Here's how the part is built. I have some questions about the finished solid (model axes, mm). A direction names the side the tool comes from. Coordinates: 2 decimals unless noted, no trailing zeros. Loops run counter-clockwise (first coordinate to the right, second up) from the corner with the lowest first, then second, coordinate; pieces in that order, holes last. Notation, with made-up numbers: (78, 20) - (117, 20) arc R18 ccw to (117, 51) - close; hole circle Ø7 at (-21, 80.25). An arc over 180 degrees is marked (long way). Use a Markdown table: item, result.
```python
from build123d import *

# Parameters (mm, degrees)
SKETCH1_W           = 335.5
SKETCH1_H           = 193
BOSS_EXTRUDE1_DEPTH = 1.5
BOSS_EXTRUDE2_DEPTH = 2
BOSS_EXTRUDE3_DEPTH = 4
SKETCH5_R           = 4
CUT_EXTRUDE1_DEPTH  = 4
SKETCH6_R           = 1.9
CUT_EXTRUDE2_DEPTH  = 14


with BuildPart() as part:
    # Sketch1 → Boss-Extrude1 (new body)
    with BuildSketch(Plane.XY):
        Rectangle(SKETCH1_W, SKETCH1_H)
    extrude(amount=BOSS_EXTRUDE1_DEPTH)

    # Sketch2 → Boss-Extrude2 (add)
    with BuildSketch(Plane.XY.offset(1.5)):
        with BuildLine():
            Line((-153.75, -90.5), (-153.75, -94.5))
            Line((-153.75, -94.5), (-6, -94.5))
            Line((-6, -94.5), (-6, -88.4))
            ThreePointArc((-6, -88.4), (-4.271930009, -84.228069991), (-0.1, -82.5))
            Line((-0.1, -82.5), (0.1, -82.5))
            ThreePointArc((0.1, -82.5), (4.271930009, -84.228069991), (6, -88.4))
            Line((6, -88.4), (6, -94.5))
            Line((6, -94.5), (153.75, -94.5))
            Line((153.75, -94.5), (153.75, -90.5))
            ThreePointArc((153.75, -90.5), (156.093145751, -84.843145751), (161.75, -82.5))
            Line((161.75, -82.5), (165.75, -82.5))
            Line((165.75, -82.5), (165.75, 82.5))
            Line((165.75, 82.5), (161.75, 82.5))
            ThreePointArc((161.75, 82.5), (156.093145751, 84.843145751), (153.75, 90.5))
            Line((153.75, 90.5), (153.75, 94.5))
            Line((153.75, 94.5), (6, 94.5))
            Line((6, 94.5), (-6, 94.5))
            Line((-6, 94.5), (-153.75, 94.5))
            Line((-153.75, 94.5), (-165.75, 94.5))
            Line((-165.75, 94.5), (-165.75, 82.5))
            Line((-165.75, 82.5), (-165.75, -82.5))
            Line((-165.75, -82.5), (-161.75, -82.5))
            ThreePointArc((-161.75, -82.5), (-156.093145751, -84.843145751), (-153.75, -90.5))
        make_face()
    extrude(amount=BOSS_EXTRUDE2_DEPTH)

    # Sketch4 → Boss-Extrude3 (add)
    with BuildSketch(Plane.XY.offset(1.5)):
        with BuildLine():
            Line((-165.75, -82.5), (-165.75, -94.5))
            Line((-165.75, -94.5), (-153.75, -94.5))
            Line((-153.75, -94.5), (-153.75, -90.5))
            ThreePointArc((-153.75, -90.5), (-156.093145751, -84.843145751), (-161.75, -82.5))
            Line((-161.75, -82.5), (-165.75, -82.5))
        make_face()
        with BuildLine():
            Line((-6, -94.5), (6, -94.5))
            Line((6, -94.5), (6, -88.4))
            ThreePointArc((6, -88.4), (4.271930009, -84.228069991), (0.1, -82.5))
            Line((0.1, -82.5), (-0.1, -82.5))
            ThreePointArc((-0.1, -82.5), (-4.271930009, -84.228069991), (-6, -88.4))
            Line((-6, -88.4), (-6, -94.5))
        make_face()
        with BuildLine():
            Line((153.75, -94.5), (165.75, -94.5))
            Line((165.75, -94.5), (165.75, -82.5))
            Line((165.75, -82.5), (161.75, -82.5))
            ThreePointArc((161.75, -82.5), (156.093145751, -84.843145751), (153.75, -90.5))
            Line((153.75, -90.5), (153.75, -94.5))
        make_face()
        with BuildLine():
            Line((165.75, 94.5), (165.75, 82.5))
            Line((165.75, 82.5), (161.75, 82.5))
            ThreePointArc((161.75, 82.5), (156.093145751, 84.843145751), (153.75, 90.5))
            Line((153.75, 90.5), (153.75, 94.5))
            Line((153.75, 94.5), (165.75, 94.5))
        make_face()
        with BuildLine():
            Line((-165.75, 24.6), (-165.75, 12.6))
            Line((-165.75, 12.6), (-159.65, 12.6))
            ThreePointArc((-159.65, 12.6), (-153.65, 18.6), (-159.65, 24.6))
            Line((-159.65, 24.6), (-165.75, 24.6))
        make_face()
        with BuildLine():
            Line((-83.85, 94.5), (-95.85, 94.5))
            Line((-95.85, 94.5), (-95.85, 88.4))
            ThreePointArc((-95.85, 88.4), (-94.121930009, 84.228069991), (-89.95, 82.5))
            Line((-89.95, 82.5), (-89.75, 82.5))
            ThreePointArc((-89.75, 82.5), (-85.578069991, 84.228069991), (-83.85, 88.4))
            Line((-83.85, 88.4), (-83.85, 94.5))
        make_face()
        with BuildLine():
            Line((46.25, 94.5), (34.25, 94.5))
            Line((34.25, 94.5), (34.25, 88.4))
            ThreePointArc((34.25, 88.4), (40.25, 82.4), (46.25, 88.4))
            Line((46.25, 88.4), (46.25, 94.5))
        make_face()
    extrude(amount=BOSS_EXTRUDE3_DEPTH)

    # Sketch5 → Cut-Extrude1 (cut)
    with BuildSketch(Plane(origin=(0, 0, 0), x_dir=(-1, 0, 0), z_dir=(0, 0, -1))):
        with Locations((-159.75, 88.5)):
            Circle(SKETCH5_R)
        with Locations((0, -88.5)):
            Circle(SKETCH5_R)
        with Locations((159.75, -88.5)):
            Circle(SKETCH5_R)
        with Locations((-159.75, -88.5)):
            Circle(SKETCH5_R)
        with Locations((89.75, 88.5)):
            Circle(SKETCH5_R)
        with Locations((-40.25, 88.4)):
            Circle(SKETCH5_R)
        with Locations((159.75, 18.6)):
            Circle(SKETCH5_R)
    extrude(amount=-CUT_EXTRUDE1_DEPTH, mode=Mode.SUBTRACT)

    # Sketch6 → Cut-Extrude2 (cut)
    with BuildSketch(Plane(origin=(0, 0, 0), x_dir=(-1, 0, 0), z_dir=(0, 0, -1))):
        with Locations((-159.75, -88.5)):
            Circle(SKETCH6_R)
        with Locations((0, -88.5)):
            Circle(SKETCH6_R)
        with Locations((159.75, -88.5)):
            Circle(SKETCH6_R)
        with Locations((-159.75, 88.5)):
            Circle(SKETCH6_R)
        with Locations((89.75, 88.5)):
            Circle(SKETCH6_R)
        with Locations((159.75, 18.6)):
            Circle(SKETCH6_R)
        with Locations((-40.25, 88.4)):
            Circle(SKETCH6_R)
    extrude(amount=-CUT_EXTRUDE2_DEPTH, mode=Mode.SUBTRACT)


solid = part.part
```
Q1. Please list where these lines run through material, in increasing order: L1, parallel to Y at x = -159.75, z = 2.7; L2, parallel to Y at x = 40.25, z = 2.9; L3, parallel to Y at x = 159.75, z = 5.25. Write a range as from..to.
Check values:
| item | result |
|---|---|
| L1 | -94.5..-92.5, -84.5..14.6, 22.6..94.5 |
| L2 | -94.5..84.4, 92.4..94.5 |
| L3 | -94.5..-90.4, -86.6..-82.75, 82.75..86.6, 90.4..94.5 |
Q2. I want a section at C-C, the plane x = -128.5. Write out the boundary of the cut face in (y, z).
Check values:
| item | result |
|---|---|
| outline | (-96.5, 0) - (96.5, 0) - (96.5, 1.5) - (94.5, 1.5) - (94.5, 3.5) - (-94.5, 3.5) - (-94.5, 1.5) - (-96.5, 1.5) - close |
Q3. Which directions (+Z, -Z, +X, -X, +Y, -Y) give clear straight access to the entire face, cutting with the end or side of a thin tool? Please do faces 5 (the face through (-85.624, 84.182, 4.486)), 6 (the face through (-161.596, -92.049, 1.972)), 7 (the face through (156.156, 84.781, 4.486)).
Check values:
| item | result |
|---|---|
| face 5 | +Z, -Y |
| face 6 | -Z |
| face 7 | +Z |
Q4. If we mould it in two halves opening along Y, with no side actions, what happens to faces 1 (the face through (-163, -88, 5.5)), 2 (the face through (4.318, -84.274, 4.486)), 3 (the face through (-2, -89, 4)), 4 (the face through (-94.168, 84.274, 4.486))? For each: pulls with the +Y half, pulls with the -Y half, needs draft (parallel to the pull), parting line crosses it, or undercut.
Check values:
| item | result |
|---|---|
| face 1 | needs draft |
| face 2 | pulls with the +Y half |
| face 3 | undercut |
| face 4 | pulls with the -Y half |
Q5. I want a section at B-B, the plane y = 30. Write out the boundary of the cut face in (x, z).
Check values:
| item | result |
|---|---|
| outline | (-167.75, 0) - (167.75, 0) - (167.75, 1.5) - (165.75, 1.5) - (165.75, 3.5) - (-165.75, 3.5) - (-165.75, 1.5) - (-167.75, 1.5) - close |
Q6. I want a section at A-A, the plane z = 2.65. Write out the boundary of the cut face in (x, y).
Check values:
| item | result |
|---|---|
| outline | (-165.75, -94.5) - (165.75, -94.5) - (165.75, 94.5) - (-165.75, 94.5) - close; hole circle Ø8 at (-159.75, -88.5); hole circle Ø8 at (-159.75, 18.6); hole circle Ø8 at (-89.75, 88.5); hole circle Ø8 at (0, -88.5); hole circle Ø8 at (40.25, 88.4); hole circle Ø8 at (159.75, -88.5); hole circle Ø8 at (159.75, 88.5) |
Q7. Will these pins go through, and if not, where does the flat tip stop? P1, Ø1, axis at x = -164, z = 4.5, coming from the +Y side; P2, Ø5, axis at x = -159.75, y = 18.6, coming from the -Z side; P3, Ø2, axis at y = -92.5, z = 5, coming from the +X side.
Check values:
| item | result |
|---|---|
| P1 | y = 24.6 |
| P2 | z = 4 |
| P3 | x = 165.75 |
